Geometry check sheet. Reference: the model listing, model coordinates, mm. Face numbers are marked on the shaded views. A direction names the side the tool comes from. Round coordinates to 2 decimals unless told otherwise and drop trailing zeros. Write each loop counter-clockwise with the first axis right and the second up, starting at its lowest first coordinate (ties: lowest second). Pieces come first, ordered by that corner, then holes. Notation, with made-up numbers: (65, -27) -> (107, -27) arc R30 ccw to (107, 6) -> close; hole circle Ø2 at (87.25, 70.5). An arc over 180 degrees is marked (long way). Use a Markdown table: item, result.
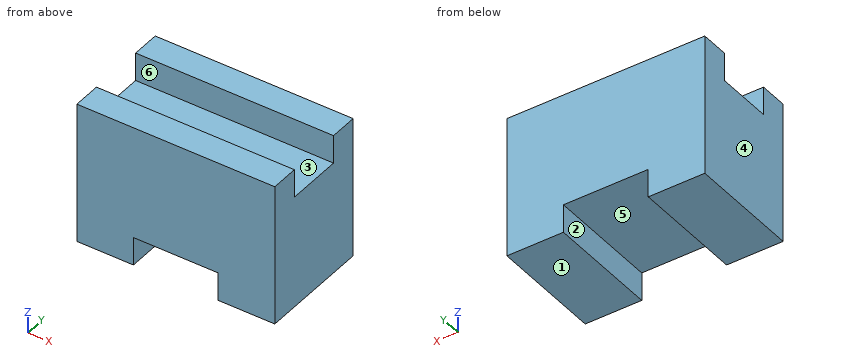
```python
from build123d import *

# Parameters (mm, degrees)
F0_W     = 25.4
F0_H     = 31.75
F1_DEPTH = 44.45
F2_W     = 44.45
F2_H     = 12.7
F3_DEPTH = 6.35
F4_W     = 19.05
F4_H     = 6.35
F5_DEPTH = 25.4


with BuildPart() as f1:
    # F0 (on Right) → F1 (new body)
    with BuildSketch(Plane.YZ):
        with Locations((-12.7, 15.875)):
            Rectangle(F0_W, F0_H)
    extrude(amount=-F1_DEPTH)

    # F2 (on face) → F3 (cut)
    with BuildSketch(Plane.XY.offset(31.75)):
        with Locations((-22.225, -12.7)):
            Rectangle(F2_W, F2_H)
    extrude(amount=-F3_DEPTH, mode=Mode.SUBTRACT)

    # F4 (on face) → F5 (cut)
    with BuildSketch(Plane.XZ.offset(25.4)):
        with Locations((-22.225, 3.175)):
            Rectangle(F4_W, F4_H)
    extrude(amount=-F5_DEPTH, mode=Mode.SUBTRACT)


solid = f1.part
```
(1) Release check for a two-part mould opening along X. For the marked faces 4, 5 and 6 record: +X half, -X half, draft (parallel to the pull), parting line (faces both ways), or undercut.
A:
| item | result |
|---|---|
| face 4 | -X half |
| face 5 | undercut |
| face 6 | draft |
(2) Thickness scan on line 1 (Y direction, x = -34, z = 30.5); line 2 (X direction, y = -8, z = 2.5); line 3 (Z direction, x = -37, y = -10). Record the ranges inside material, lowest first.
A:
| item | result |
|---|---|
| line 1 | y = -25.4 to -19.05, -6.35 to 0 |
| line 2 | x = -44.45 to -31.75, -12.7 to 0 |
| line 3 | z = 0 to 25.4 |
(3) Section check C-C on x = -38.5. Record the cut outline in (y, z).
A:
| item | result |
|---|---|
| outline | (-25.4, 0) -> (0, 0) -> (0, 31.75) -> (-6.35, 31.75) -> (-6.35, 25.4) -> (-19.05, 25.4) -> (-19.05, 31.75) -> (-25.4, 31.75) -> close |
(4) Gauge pin test, flat ends, axial feed: pin 1 Ø9.5 at (x, y) = (-19.5, -10) entering from -Z; pin 2 Ø5 at (x, y) = (-29.5, -12.5) entering from +Z. Record the tip position at first contact, or that the pin passes through.
A:
| item | result |
|---|---|
| pin 1 | stops at z = 6.35 |
| pin 2 | stops at z = 25.4 |
(5) Section check A-A on z = 28. Record the cut outline in (x, y), plus the area to 3 significant figures.
A:
| item | result |
|---|---|
| outline | (-44.45, -25.4) -> (0, -25.4) -> (0, -19.05) -> (-44.45, -19.05) -> close; (-44.45, -6.35) -> (0, -6.35) -> (0, 0) -> (-44.45, 0) -> close |
| area | 565 mm2 |
(6) Access from +Z, -Z, +X, -X, +Y, -Y to the whole of each face (thin tool, end or side, straight path). Record for the marked faces 1, 2 and 3.
A:
| item | result |
|---|---|
| face 1 | -Z, +X, -X, +Y, -Y |
| face 2 | -Z, +Y, -Y |
| face 3 | +Z, +X, -X |
(7) Section check B-B on y = -21.75. Record the cut outline in (x, z).
A:
| item | result |
|---|---|
| outline | (-44.45, 0) -> (-31.75, 0) -> (-31.75, 6.35) -> (-12.7, 6.35) -> (-12.7, 0) -> (0, 0) -> (0, 31.75) -> (-44.45, 31.75) -> close |
